The listing builds one solid part. Answer for the finished solid, in the listing's coordinates (mm). A direction names the side the tool comes from. Coordinates: 2 decimals unless noted, no trailing zeros. Order: outer loops, then holes, each group sorted by start corner. A loop starts at its lowest first (then second) coordinate and runs counter-clockwise, first axis right, second up.
```python
from build123d import *

# Parameters (mm, degrees)
SKETCH_1_R      = 5.75
SKETCH_1_R_2    = 2.83
EXTRUDE_1_DEPTH = 11
SKETCH_2_R      = 26.8
EXTRUDE_2_DEPTH = 1.5
EXTRUDE_START   = 1.5
SKETCH_3_R      = 26.8
SKETCH_3_R_2    = 24.8
EXTRUDE_3_DEPTH = 1.5
SKETCH_4_R      = 0.85


with BuildPart() as part:
    # Эскиз1 → Бобышка-Вытянуть1 (new body)
    # profile 1 of 3: a face of its own
    with BuildSketch(Plane.XY):
        Circle(SKETCH_1_R)
        Circle(SKETCH_1_R_2, mode=Mode.SUBTRACT)
    # profile 2 of 3: a face of its own
    with BuildSketch(Plane.XY):
        with BuildLine():
            ThreePointArc((2.002223764, 2), (0, 2.83), (-2.002223764, 2))
            Line((-2.002223764, 2), (2.002223764, 2))
        make_face()
    # profile 3 of 3: a face of its own
    with BuildSketch(Plane.XY):
        with BuildLine():
            Line((2.002223764, -2), (-2.002223764, -2))
            ThreePointArc((-2.002223764, -2), (0, -2.83), (2.002223764, -2))
        make_face()
    extrude(amount=EXTRUDE_1_DEPTH)

    # Эскиз2 → Бобышка-Вытянуть2 (add)
    with BuildSketch(Plane.XY.offset(11)):
        Circle(SKETCH_2_R)
    extrude(amount=EXTRUDE_2_DEPTH)

    # Эскиз3 → Бобышка-Вытянуть3 (add)
    with BuildSketch(Plane(origin=(0, 0, 11), x_dir=(-1, 0, 0), z_dir=(0, 0, -1)).offset(EXTRUDE_START)):
        Circle(SKETCH_3_R)
        Circle(SKETCH_3_R_2, mode=Mode.SUBTRACT)
    extrude(amount=-EXTRUDE_3_DEPTH)

    # Эскиз4 → Вырез-Повернуть1 (revolve, cut)
    with BuildSketch(Plane(origin=(0, 0, 0), x_dir=(0, 0, -1), z_dir=(1, 0, 0)), mode=Mode.PRIVATE) as cut_revolve_1_sk:
        with Locations((-11, 26.8)):
            Circle(SKETCH_4_R)
    revolve(cut_revolve_1_sk.sketch.rotate(Axis((0, 0, 11), (0, 0, -1)), 270), axis=Axis((0, 0, 11), (0, 0, -1)), mode=Mode.SUBTRACT)


solid = part.part
```
(1) For faces 4 (the face through (26.774, 1.178, 9.82)), 5 (the face through (0, -2, 5)), determine the directions among +Z, -Z, +X, -X, +Y, -Y from which every point of the face is accessible in a straight line to the end or side of a thin tool.
(2) Find section C-C (z = 8.25). Write down the section's boundary in (x, y).
(3) Consider line 1 (Y direction, x = 0, z = 9.9); line 2 (Y direction, x = 0, z = 10.25); line 3 (X direction, y = 5, z = 8). Determine where each line is inside the solid, lowest interval first.
(4) Find section B-B (x = 0). Write down the section's boundary in (y, z).
(5) The mould has two halves that part along X. Classify faces 1 (the face through (-21.268, -16.307, 12.17)), 2 (the face through (0, 0, 11)), 3 (the face through (0, 0, 12.5)): released by +X, released by -X, zero draft, split by the parting line, or undercut.
(6) Each of these flat-tipped pins is pushed along its axis until it touches: pin 1 Ø1.5 at (y, z) = (-3, 4.5) entering from +X; pin 2 Ø2 at (y, z) = (-12, 9) entering from -X; pin 3 Ø4.5 at (x, z) = (-0.5, 7) entering from -Y. Where does it stop, or does it pass through?
(7) Find section A-A (y = 0). Write down the section's boundary in (x, z), and give its area (3 significant figures).
Findings below:
1. face 4: +Z, -Z
1. face 5: -Z
2. outline: circle Ø11.5 at (0, 0); hole (-2, -2) - (2, -2) arc R2.83 ccw to (2, 2) - (-2, 2) arc R2.83 ccw to start
3. line 1: y = -26.8 to -24.8, -5.75 to -2, 2 to 5.75, 24.8 to 26.8
3. line 2: y = -26.4 to -24.8, -5.75 to -2, 2 to 5.75, 24.8 to 26.4
3. line 3: x = -2.84 to 2.84
4. outline: (-26.8, 9.5) - (-24.8, 9.5) - (-24.8, 11) - (-5.75, 11) - (-5.75, 0) - (-2, 0) - (-2, 11) - (2, 11) - (2, 0) - (5.75, 0) - (5.75, 11) - (24.8, 11) - (24.8, 9.5) - (26.8, 9.5) - (26.8, 10.15) arc R0.85 cw to (26.8, 11.85) - (26.8, 12.5) - (-26.8, 12.5) - (-26.8, 11.85) arc R0.85 cw to (-26.8, 10.15) - close
5. face 1: split by the parting line
5. face 2: undercut
5. face 3: zero draft
6. pin 1: stops at x = 5.29
6. pin 2: stops at x = -24.38
6. pin 3: stops at y = -5.75
7. outline: (-26.8, 9.5) - (-24.8, 9.5) - (-24.8, 11) - (-5.75, 11) - (-5.75, 0) - (-2.83, 0) - (-2.83, 11) - (2.83, 11) - (2.83, 0) - (5.75, 0) - (5.75, 11) - (24.8, 11) - (24.8, 9.5) - (26.8, 9.5) - (26.8, 10.15) arc R0.85 cw to (26.8, 11.85) - (26.8, 12.5) - (-26.8, 12.5) - (-26.8, 11.85) arc R0.85 cw to (-26.8, 10.15) - close
7. area: 148 mm2
